Model file for the job. Use its own axes, mm. A direction names the side the tool comes from. Round coordinates to 2 decimals unless told otherwise and drop trailing zeros. Order: outer loops, then holes, each group sorted by start corner. A loop starts at its lowest first (then second) coordinate and runs counter-clockwise, first axis right, second up. Notation, with made-up numbers: (25.25, 31) - (41.25, 31) arc R21 ccw to (41.25, 62) - close; hole circle Ø11 at (-39.75, 71). An arc over 180 degrees is marked (long way). Put each result on its own line as item: value. Start each with the question number.
Item 1: Saw through at A-A on x = 67. List the corners of the cut face in (y, z), plus the area to 3 significant figures.
Item 2: Probe probe 1 along Z at (x, y) = (-90, 14); probe 2 along X at (y, z) = (63, 14.5); probe 3 along Y at (x, z) = (1, 4). List the from-to ranges inside material, lowest first.
Item 3: Mould opens along Y. For faces 6 (the face through (69.07, 81, 0.03)), 7 (the face through (-5, 53.841, 17)), 8 (the face through (-5, 61, 30.595)) say: pulls with the +Y half, pulls with the -Y half, needs draft (parallel to the pull), parting line crosses it, or undercut.
Item 4: Saw through at D-D on x = -41. List the corners of the cut face in (y, z), plus the area to 3 significant figures.
Item 5: Saw through at C-C on y = 64.5. List the corners of the cut face in (x, z).
Item 6: Pin check, flat tips, straight feed: pin 1 Ø6 at (x, y) = (66.44, 76.88) entering from -Z; pin 2 Ø1.5 at (x, y) = (18.5, 11.5) entering from +Z; pin 3 Ø3.5 at (x, z) = (6.5, 14.5) entering from -Y; pin 4 Ø4 at (y, z) = (60.5, 10.5) entering from -X. Stop position of each tip, or through.
Item 7: Which spindle directions (+Z, -Z, +X, -X, +Y, -Y) get a long thin tool onto all of the face, cutting with end or side? Do faces 1 (the face through (5, 67.562, 16)), 2 (the face through (-10.9, 61, 16)), 3 (the face through (11, 61, 17)), 4 (the face through (5, 53.841, 16)), 5 (the face through (-1, 47, -2.41)). Say none if no direction does.
```python
from build123d import *

# Parameters (mm, degrees)
F0_W      = 203.408972
F0_H      = 4.820996
F1_DEPTH  = 95.25
F2_W      = 13.721295
F2_H      = 30.594785
F3_DEPTH  = 11
F3_FACE_W = 13.721294
F3_FACE_H = 28.184286
F4_DEPTH  = 10.9
F5_R      = 4.891712
F6_DEPTH  = 4.821996


with BuildPart() as f1:
    # F0 (on Front) → F1 (new body)
    with BuildSketch(Plane.XZ):
        Rectangle(F0_W, F0_H)
    extrude(amount=-F1_DEPTH)

    # F2 (on Right) → F3 (join)
    with BuildSketch(Plane.YZ):
        with Locations((60.701731, 15.297392)):
            Rectangle(F2_W, F2_H)
    extrude(amount=F3_DEPTH)

    # F3_face (on face) → F4 (join)
    with BuildSketch(Plane(origin=(0, 60.701732, 16.502641), x_dir=(0, 1, 0), z_dir=(-1, 0, 0))):
        Rectangle(F3_FACE_W, F3_FACE_H)
    extrude(amount=F4_DEPTH)

    # F5 (on face) → F6 (cut, through all)
    with BuildSketch(Plane.XY.offset(2.410498)):
        with Locations((66.436283, 76.876432)):
            Circle(F5_R)
        with Locations((49.508363, 76.876432)):
            Circle(F5_R)
    extrude(amount=-F6_DEPTH, mode=Mode.SUBTRACT)


solid = f1.part
```
Results found:
1. outline: (0, -2.41) - (72.02, -2.41) - (72.02, 2.41) - (0, 2.41) - close; (81.74, -2.41) - (95.25, -2.41) - (95.25, 2.41) - (81.74, 2.41) - close
1. area: 412 mm²
2. probe 1: z = -2.41 to 2.41
2. probe 2: x = -10.9 to 11
2. probe 3: y = 53.84 to 67.56
3. face 6: undercut
3. face 7: pulls with the -Y half
3. face 8: needs draft
4. outline: (0, -2.41) - (95.25, -2.41) - (95.25, 2.41) - (0, 2.41) - close
4. area: 459 mm²
5. outline: (-101.7, -2.41) - (101.7, -2.41) - (101.7, 2.41) - (11, 2.41) - (11, 30.59) - (-10.9, 30.59) - (-10.9, 2.41) - (-101.7, 2.41) - close
6. pin 1: passes through
6. pin 2: stops at z = 2.41
6. pin 3: stops at y = 53.84
6. pin 4: stops at x = -10.9
7. face 1: +Z, +X, -X, +Y
7. face 2: +Z, -X, +Y, -Y
7. face 3: +Z, +X, +Y, -Y
7. face 4: +Z, +X, -X, -Y
7. face 5: -Z, +X, -X, +Y, -Y
